CAD build for the part. Positions are in the model's coordinates, mm. Face numbers are marked on the shaded views. A direction names the side the tool comes from. Coordinates: 2 decimals unless noted, no trailing zeros. Loops run counter-clockwise (first coordinate to the right, second up) from the corner with the lowest first, then second, coordinate; pieces in that order, holes last.
1) Which spindle directions (+Z, -Z, +X, -X, +Y, -Y) get a long thin tool onto all of the face, cutting with end or side? Do the marked faces 1, 2, 3, 4 and 5. Say none if no direction does.
2) Saw through at C-C, the plane x = 45. Write the cut outline in (y, z).
3) Two-plate mould, pull along X, no slides. Class the marked faces 6, 7, 8 and 9: +X half, -X half, draft (parallel to the pull), parting line (faces both ways), or undercut.
4) Saw through at A-A, the plane x = 10. Write the cut outline in (y, z), and give its area (3 significant figures).
5) Saw through at B-B, the plane z = 1. Give the number of separate pieces and of enclosed holes in the cut face, and give its area (3 significant figures).
6) Pin check, flat tips, straight feed: pin 1 Ø6 at (x, y) = (64.5, 30.5) entering from -Z; pin 2 Ø1.5 at (y, z) = (16.5, 1.5) entering from +X; pin 3 Ø3 at (y, z) = (28.5, 2.5) entering from -X. Stop position of each tip, or through.
7) Wall check: line 1 along Y through (x, z) = (64.5, 3.95); line 2 along Y through (x, z) = (64.5, 2.1); line 3 along Y through (x, z) = (29.5, 3.25). Give the ranges that are in metal, low to high.
```python
from build123d import *

# Parameters (mm, degrees)
SKETCH1_R           = 1.5
BOSS_EXTRUDE1_DEPTH = 6
SKETCH2_R           = 3.25
CUT_EXTRUDE1_DEPTH  = 3
FILLET1_R           = 2.5
FILLET2_R           = 1.5
FILLET3_R           = 10
CUT_EXTRUDE2_DEPTH  = 2
SKETCH4_R           = 1.35
CUT_EXTRUDE3_DEPTH  = 7
CUT_EXTRUDE4_START  = -10
SKETCH5_R           = 1.35
CUT_EXTRUDE4_DEPTH  = 10


with BuildPart() as part:
    # Sketch1 → Boss-Extrude1 (new body)
    with BuildSketch(Plane.XY):
        Polygon((2.5, 35), (69, 35), (69, 18), (62, 18), (62, 0), (0, 0), (0, 3.474843555), (7.106575765, 23), (2.5, 23), align=None)
        with Locations((64.5, 30.5)):
            Circle(SKETCH1_R, mode=Mode.SUBTRACT)
        with Locations((64.5, 21.5)):
            Circle(SKETCH1_R, mode=Mode.SUBTRACT)
        with BuildLine():
            Line((58.25, 20.5), (58.25, 13))
            ThreePointArc((58.25, 13), (52, 6.75), (45.75, 13))
            Line((45.75, 13), (45.75, 20.5))
            ThreePointArc((45.75, 20.5), (52, 26.75), (58.25, 20.5))
        make_face(mode=Mode.SUBTRACT)
        Polygon((7.5, 8), (39.75, 8), (39.75, 23), (12.959553514, 23), align=None, mode=Mode.SUBTRACT)
        with BuildLine():
            Line((16.959553514, 30), (31.75, 30))
            ThreePointArc((31.75, 30), (33.5, 28.25), (31.75, 26.5))
            Line((31.75, 26.5), (16.959553514, 26.5))
            ThreePointArc((16.959553514, 26.5), (15.209553514, 28.25), (16.959553514, 30))
        make_face(mode=Mode.SUBTRACT)
        with BuildLine():
            Line((16.959553514, 1.5), (31.75, 1.5))
            ThreePointArc((31.75, 1.5), (33.5, 3.25), (31.75, 5))
            Line((31.75, 5), (16.959553514, 5))
            ThreePointArc((16.959553514, 5), (15.209553514, 3.25), (16.959553514, 1.5))
        make_face(mode=Mode.SUBTRACT)
    extrude(amount=BOSS_EXTRUDE1_DEPTH)

    # Sketch2 → Cut-Extrude1 (cut)
    with BuildSketch(Plane(origin=(0, 0, 0), x_dir=(-1, 0, 0), z_dir=(0, 0, -1))):
        with Locations((-64.5, 30.5)):
            Circle(SKETCH2_R)
        with Locations((-64.5, 21.5)):
            Circle(SKETCH2_R)
        with BuildLine():
            Line((-44.3, 20.5), (-44.3, 13))
            ThreePointArc((-44.3, 13), (-52, 5.3), (-59.7, 13))
            Line((-59.7, 13), (-59.7, 20.5))
            ThreePointArc((-59.7, 20.5), (-52, 28.2), (-44.3, 20.5))
        make_face()
    extrude(amount=-CUT_EXTRUDE1_DEPTH, mode=Mode.SUBTRACT)

    # Fillet1
    fillet1_edges = [part.edges().sort_by_distance(p)[0] for p in [
        (0, 0, 3),
        (0, 3.474843555, 3),
        (2.5, 23, 3),
        (2.5, 35, 3),
        (69, 35, 3),
        (69, 18, 3),
        (62, 18, 3),
        (12.959553514, 23, 3),
        (7.5, 8, 3),
        (39.75, 8, 3),
        (39.75, 23, 3),
    ]]
    fillet(fillet1_edges, radius=FILLET1_R)

    # Fillet2
    fillet2_edges = [part.edges().sort_by_distance(p)[0] for p in [
        (7.106575765, 23, 3),
    ]]
    fillet(fillet2_edges, radius=FILLET2_R)

    # Fillet3
    fillet3_edges = [part.edges().sort_by_distance(p)[0] for p in [
        (62, 0, 3),
    ]]
    fillet(fillet3_edges, radius=FILLET3_R)

    # Sketch3 → Cut-Extrude2 (cut)
    with BuildSketch(Plane(origin=(0, 0, 0), x_dir=(-1, 0, 0), z_dir=(0, 0, -1))):
        with BuildLine():
            Line((-31.75, 31.75), (-16.959553514, 31.75))
            ThreePointArc((-16.959553514, 31.75), (-13.459553514, 28.25), (-16.959553514, 24.75))
            Line((-16.959553514, 24.75), (-31.75, 24.75))
            ThreePointArc((-31.75, 24.75), (-35.25, 28.25), (-31.75, 31.75))
        make_face()
        with BuildLine():
            Line((-31.75, 6.75), (-16.959553514, 6.75))
            ThreePointArc((-16.959553514, 6.75), (-14.48467978, 5.724873734), (-13.459553514, 3.25))
            Line((-13.459553514, 3.25), (-13.459553514, 0))
            Line((-13.459553514, 0), (-35.25, 0))
            Line((-35.25, 0), (-35.25, 3.25))
            ThreePointArc((-35.25, 3.25), (-34.224873734, 5.724873734), (-31.75, 6.75))
        make_face()
    extrude(amount=-CUT_EXTRUDE2_DEPTH, mode=Mode.SUBTRACT)

    # Sketch4 → Cut-Extrude3 (cut)
    with BuildSketch(Plane.XZ):
        with Locations(Location((10, 3, 0), (0, 0, 270))):
            Circle(SKETCH4_R)
        with Locations(Location((45, 3, 0), (0, 0, 270))):
            Circle(SKETCH4_R)
    extrude(amount=-CUT_EXTRUDE3_DEPTH, mode=Mode.SUBTRACT)

    # Sketch5 → Cut-Extrude4 (cut)
    with BuildSketch(Plane(origin=(0, 35, 0), x_dir=(1, 0, 0), z_dir=(0, 1, 0)).offset(CUT_EXTRUDE4_START)):
        with Locations(Location((10, -3, 0), (0, 0, 90))):
            Circle(SKETCH5_R)
    extrude(amount=CUT_EXTRUDE4_DEPTH, mode=Mode.SUBTRACT)


solid = part.part
```
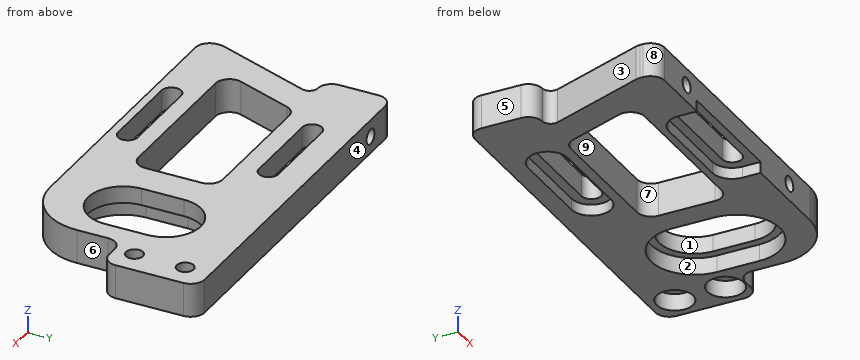
Data:
1. face 1: +Z, -Z
1. face 2: -Z
1. face 3: +Z, -Z, -X
1. face 4: +Z, -Z, +X, -X, +Y
1. face 5: +Z, -Z, -X, +Y
2. outline: (0, 0) - (9.79, 0) - (9.79, 3) - (23.71, 3) - (23.71, 0) - (35, 0) - (35, 6) - (0, 6) - (0, 4.35) - (7, 4.35) - (7, 1.65) - (0, 1.65) - close
3. face 6: +X half
3. face 7: undercut
3. face 8: -X half
3. face 9: undercut
4. outline: (0, 0) - (8.24, 0) - (8.24, 6) - (0, 6) - (0, 4.35) - (7, 4.35) - (7, 1.65) - (0, 1.65) - close; (14.87, 0) - (35, 0) - (35, 1.65) - (25, 1.65) - (25, 4.35) - (35, 4.35) - (35, 6) - (14.87, 6) - close
4. area: 124 mm2
5. separate pieces: 1
5. enclosed holes: 5
5. area: 1,080 mm2
6. pin 1: stops at z = 3
6. pin 2: stops at x = 62.71
6. pin 3: stops at x = 2.5
7. line 1: y = 18 to 20, 23 to 29, 32 to 35
7. line 2: y = 18 to 18.25, 24.75 to 27.25, 33.75 to 35
7. line 3: y = 0 to 1.5, 5 to 8, 23 to 26.5, 30 to 35
